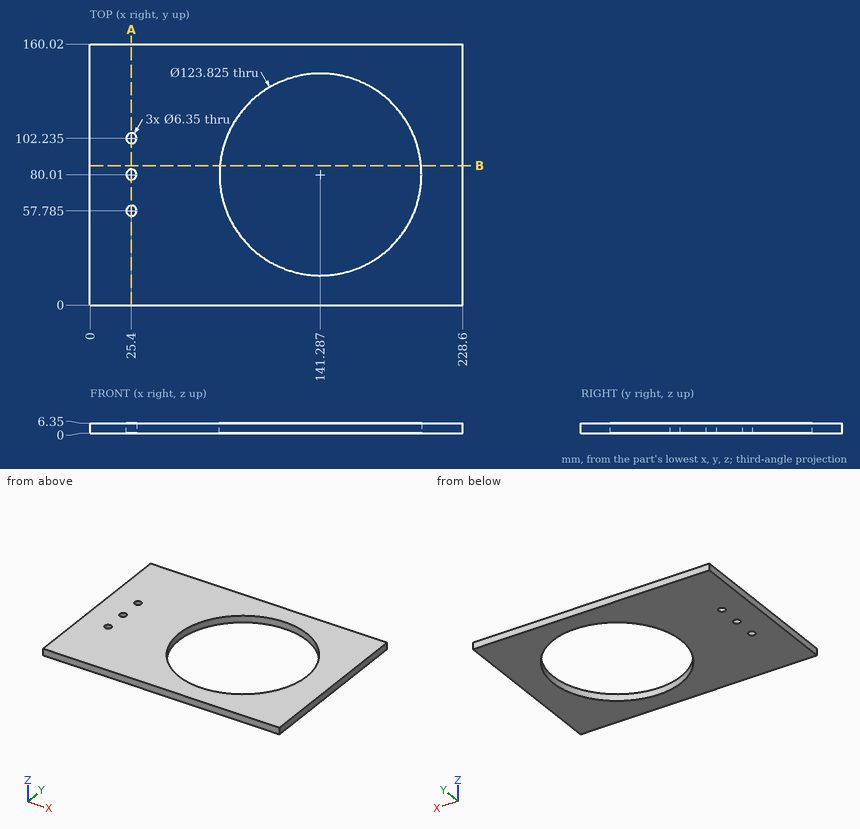
Here's the drawing with two shaded views (mm, measured from the low corner). I have some questions. Give positions to 0.01 mm unless a question says otherwise; leave off trailing zeros. Loops run counter-clockwise (first coordinate to the right, second up) from the corner with the lowest first, then second, coordinate; pieces in that order, holes last. Notation, with made-up numbers: (16, -37) -> (55, -37) arc R25 ccw to (55, -23) -> close; hole circle Ø3 at (87.5, 38.25). An arc over 180 degrees is marked (long way). Answer as a JSON object with one key per item and string values. Group by question number.
Item 1: I need wall thicknesses on L1, parallel to Y at x = 25.4, z = 4 (1 decimal); L2, parallel to Y at x = 139, z = 6; L3, parallel to X at y = 56.5, z = 2.5 (1 decimal). Which ranges of each line are inside material? Lowest first, please.
Item 2: Imagine slicing it at B-B on y = 85.5. Write out the boundary of the cut face in (x, z).
Item 3: Will this pin go through, and if not, where does the flat tip stop? pin 1 (1.5 mm diameter, centred on y = 91.5, z = 4.5, fed in from -X).
Item 4: Imagine slicing it at A-A on x = 25.4. Give the number of separate pieces and of enclosed holes in the cut face, then the cut area to 3 significant figures.
Answer list:
{
 "1": {"L1": "y = 0 to 54.6, 61 to 76.8, 83.2 to 99.1, 105.4 to 160", "L2": "y = 0 to 18.14, 141.88 to 160.02", "L3": "x = 0 to 22.5, 28.3 to 84, 198.6 to 228.6"},
 "2": {"outline": "(0, 0) -> (79.62, 0) -> (79.62, 6.35) -> (0, 6.35) -> close; (202.96, 0) -> (228.6, 0) -> (228.6, 6.35) -> (202.96, 6.35) -> close"},
 "3": {"pin 1": "stops at x = 0"},
 "4": {"separate pieces": "4", "enclosed holes": "0", "area": "895 mm2"}
}
